Here's the drawing with two shaded views (mm, measured from the low corner). I have some questions. Round coordinates to 2 decimals unless told otherwise and drop trailing zeros. Loops run counter-clockwise (first coordinate to the right, second up) from the corner with the lowest first, then second, coordinate; pieces in that order, holes last.
(1) If I drill on line 1 along X through (y, z) = (2.55, 2); line 2 along X through (y, z) = (0.75, 35.5); line 3 along X through (y, z) = (2.85, 16.5), over which ranges is the centre line in solid material (lowest first)?
(2) Will this pin go through, and if not, where does the flat tip stop? pin 1 Ø3 at (x, z) = (14.5, 35.5) entering from -Y.
(3) I want a section at A-A on z = 16.5. Write out the boundary of the cut face in (x, y).
(4) I want a section at B-B on z = 35.5. Write out the boundary of the cut face in (x, y).
(5) I want a section at C-C on z = 6. Write out the boundary of the cut face in (x, y), plus the area to 3 significant figures.
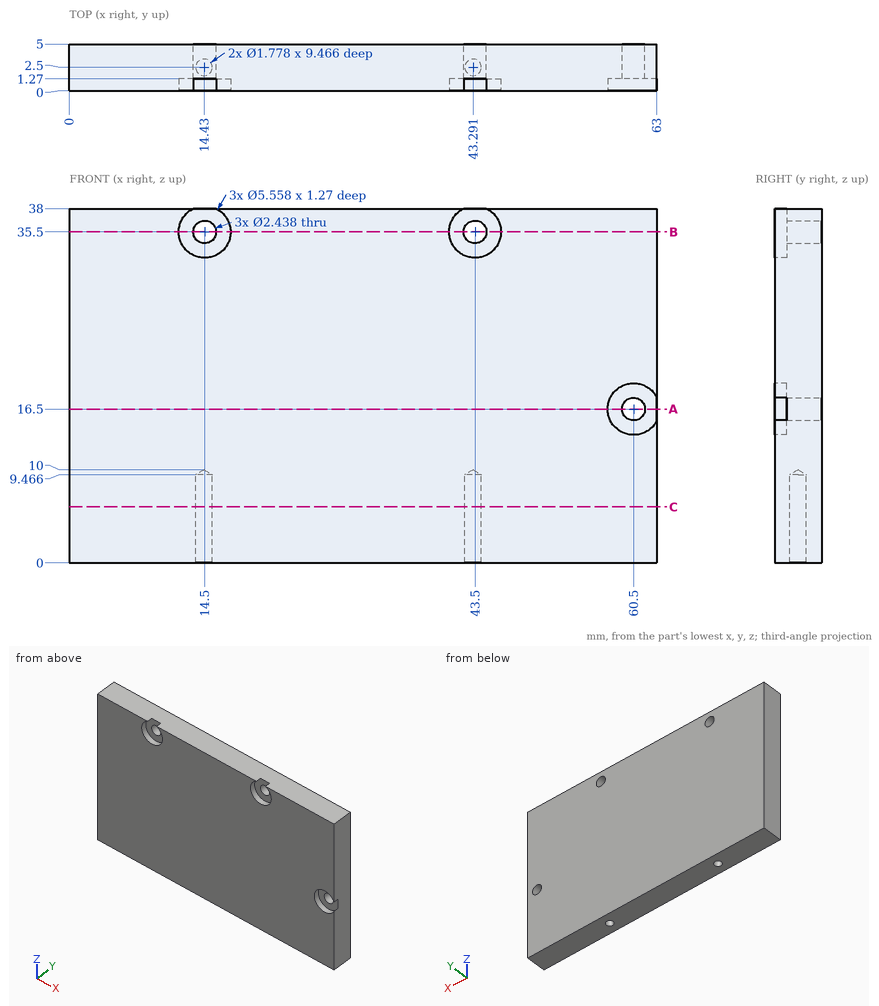
Filled sheet:
1. line 1: x = 0 to 13.54, 15.32 to 42.4, 44.18 to 63
1. line 2: x = 0 to 11.72, 17.28 to 40.72, 46.28 to 63
1. line 3: x = 0 to 59.28, 61.72 to 63
2. pin 1: stops at y = 1.27
3. outline: (0, 0) - (57.72, 0) - (57.72, 1.27) - (59.28, 1.27) - (59.28, 5) - (0, 5) - close; (61.72, 1.27) - (63, 1.27) - (63, 5) - (61.72, 5) - close
4. outline: (0, 0) - (11.72, 0) - (11.72, 1.27) - (13.28, 1.27) - (13.28, 5) - (0, 5) - close; (15.72, 1.27) - (17.28, 1.27) - (17.28, 0) - (40.72, 0) - (40.72, 1.27) - (42.28, 1.27) - (42.28, 5) - (15.72, 5) - close; (44.72, 1.27) - (46.28, 1.27) - (46.28, 0) - (63, 0) - (63, 5) - (44.72, 5) - close
5. outline: (0, 0) - (63, 0) - (63, 5) - (0, 5) - close; hole circle Ø1.78 at (14.43, 2.5); hole circle Ø1.78 at (43.29, 2.5)
5. area: 310 mm2
